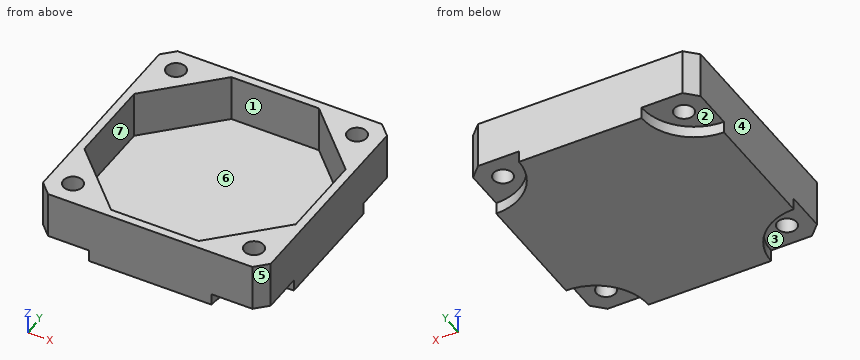
from build123d import *

# Parameters (mm, degrees)
F0_W     = 39
F0_H     = 39
F1_DEPTH = 10
F3_DEPTH = 2
F4_D     = 3.3
F4_DEPTH = 20
F4_TIP   = 0.9914200214
F5_SIZE  = 2
F8_DEPTH = 8


with BuildPart() as f1:
    # F0 (on Top) → F1 (new body)
    with BuildSketch(Plane.XY):
        with Locations((-18.7466505767, 6.1744563282)):
            Rectangle(F0_W, F0_H)
    extrude(amount=F1_DEPTH)

    # F2 (on face) → F3 (cut)
    with BuildSketch(Plane.XY):
        with BuildLine():
            ThreePointArc((-8.2466505767, 25.6744563282), (-5.6106116074, 19.3104952975), (0.7533494233, 16.6744563282))
            Line((0.7533494233, 16.6744563282), (0.7533494233, 25.6744563282))
            Line((0.7533494233, 25.6744563282), (-8.2466505767, 25.6744563282))
        make_face()
        with BuildLine():
            ThreePointArc((-38.2466505767, 16.6744563282), (-31.882689546, 19.3104952975), (-29.2466505767, 25.6744563282))
            Line((-29.2466505767, 25.6744563282), (-38.2466505767, 25.6744563282))
            Line((-38.2466505767, 25.6744563282), (-38.2466505767, 16.6744563282))
        make_face()
        with BuildLine():
            Line((-38.2466505767, -13.3255436718), (-29.2466505767, -13.3255436718))
            ThreePointArc((-29.2466505767, -13.3255436718), (-31.882689546, -6.9615826412), (-38.2466505767, -4.3255436718))
            Line((-38.2466505767, -4.3255436718), (-38.2466505767, -13.3255436718))
        make_face()
        with BuildLine():
            Line((-8.2466505767, -13.3255436718), (0.7533494233, -13.3255436718))
            Line((0.7533494233, -13.3255436718), (0.7533494233, -4.3255436718))
            ThreePointArc((0.7533494233, -4.3255436718), (-5.6106116074, -6.9615826412), (-8.2466505767, -13.3255436718))
        make_face()
    extrude(amount=F3_DEPTH, mode=Mode.SUBTRACT)

    # F4
    with Locations(Plane(origin=(0, 0, 0), x_dir=(1, 0, 0), z_dir=(0, 0, -1))):
        with Locations((-3.2466505767, -21.6744563282), (-34.2466505767, -21.6744563282), (-34.2466505767, 9.3255436718), (-3.2466505767, 9.3255436718)):
            Hole(F4_D / 2, depth=F4_DEPTH)
            with Locations((0, 0, -(F4_DEPTH + F4_TIP / 2))):  # 118° drill point
                Cone(0, F4_D / 2, F4_TIP, mode=Mode.SUBTRACT)

    # F5
    f5_edges = [f1.edges().sort_by_distance(p)[0] for p in [
        (0.753349, -13.325544, 6),
        (0.753349, 25.674456, 6),
        (-38.246651, 25.674456, 6),
        (-38.246651, -13.325544, 6),
    ]]
    chamfer(f5_edges, length=F5_SIZE)

    # F7 (on face) → F8 (cut)
    with BuildSketch(Plane.XY.offset(10)):
        Polygon((-11.2466505767, -11.9321453896), (-0.6400488589, -1.3255436718), (-0.6400488589, 13.6744563282), (-11.2466505767, 24.281058046), (-26.2466505767, 24.281058046), (-36.8532522945, 13.6744563282), (-36.8532522945, -1.3255436718), (-26.2466505767, -11.9321453896), align=None)
    extrude(amount=-F8_DEPTH, mode=Mode.SUBTRACT)


solid = f1.part
Input: part model. Units: mm. Frame: model coordinates. Face numbers are marked on the shaded views. A direction names the side the tool comes from. Give positions to 0.01 mm unless a question says otherwise; leave off trailing zeros. Order: outer loops, then holes, each group sorted by start corner. A loop starts at its lowest first (then second) coordinate and runs counter-clockwise, first axis right, second up. Notation, with made-up numbers: (0.25, 41) -> (36.25, 41) arc R19 ccw to (36.25, 50) -> close; hole circle Ø10 at (-34.75, 10). An arc over 180 degrees is marked (long way). Use one line per item in the form item = value.
1) Mould query, pull axis Y, two halves, no side actions, for the marked faces 4, 5, 6 and 7. Classes: pulls with the +Y half, pulls with the -Y half, needs draft (parallel to the pull), parting line crosses it, or undercut.
Response values:
face_4 = needs draft
face_5 = pulls with the -Y half
face_6 = undercut
face_7 = undercut
2) Section C-C, the plane y = 21. Return loops of the section in (x, z).
Response values:
outline = (-38.25, 2) -> (-35.75, 2) -> (-35.75, 10) -> (-38.25, 10) -> close; (-32.74, 2) -> (-30.56, 2) -> (-30.56, 0) -> (-6.94, 0) -> (-6.94, 2) -> (-4.75, 2) -> (-4.75, 10) -> (-7.97, 10) -> (-7.97, 2) -> (-29.53, 2) -> (-29.53, 10) -> (-32.74, 10) -> close; (-1.74, 2) -> (0.75, 2) -> (0.75, 10) -> (-1.74, 10) -> close
3) Reachability of the marked faces 1, 2 and 3 from +Z, -Z, +X, -X, +Y, -Y: full face, straight path, thin tool, end or side. Return the list, or none.
Response values:
face_1 = +Z
face_2 = -Z, -X, +Y
face_3 = -Z, -X, -Y
4) Section B-B, the plane x = -12. Return loops of the section in (y, z).
Response values:
outline = (-13.33, 0) -> (25.67, 0) -> (25.67, 10) -> (24.28, 10) -> (24.28, 2) -> (-11.93, 2) -> (-11.93, 10) -> (-13.33, 10) -> close
5) Line query: probe 1 along X at (y, z) = (-0.5, 3.5); probe 2 along Y at (x, z) = (-26, 2.75); probe 3 along Z at (x, y) = (-33.5, 15). Output: solid intervals per line, ascending.
Response values:
probe_1 = -38.25 to -36.85, -0.64 to 0.75
probe_2 = -13.33 to -11.93, 24.28 to 25.67
probe_3 = 0 to 2
6) Section A-A, the plane y = 13. Return loops of the section in (x, z).
Response values:
outline = (-38.25, 0) -> (0.75, 0) -> (0.75, 10) -> (-0.64, 10) -> (-0.64, 2) -> (-36.85, 2) -> (-36.85, 10) -> (-38.25, 10) -> close
7) First-contact query: pin 1 Ø1 at (x, y) = (-10, 21.5) entering from +Z; pin 2 Ø4.5 at (x, y) = (-34.25, 21.67) entering from +Z. Flat tips, straight axial feed; report the tip coordinate or a pass-through.
Response values:
pin_1 = 2
pin_2 = 10
8) Section D-D, the plane z = 3. Return loops of the section in (x, y).
Response values:
outline = (-38.25, -11.33) -> (-36.25, -13.33) -> (-1.25, -13.33) -> (0.75, -11.33) -> (0.75, 23.67) -> (-1.25, 25.67) -> (-36.25, 25.67) -> (-38.25, 23.67) -> close; hole (-36.85, -1.33) -> (-26.25, -11.93) -> (-11.25, -11.93) -> (-0.64, -1.33) -> (-0.64, 13.67) -> (-11.25, 24.28) -> (-26.25, 24.28) -> (-36.85, 13.67) -> close; hole circle Ø3.3 at (-34.25, -9.33); hole circle Ø3.3 at (-34.25, 21.67); hole circle Ø3.3 at (-3.25, -9.33); hole circle Ø3.3 at (-3.25, 21.67)
